Input: part model. Units: mm. Frame: model coordinates. Face numbers are marked on the shaded views. A direction names the side the tool comes from. Round coordinates to 2 decimals unless told otherwise and drop trailing zeros. Order: outer loops, then holes, each group sorted by start corner. A loop starts at its lowest first (then second) coordinate and runs counter-clockwise, first axis right, second up.
Item 1: Cut plane A-A on z = 0. Output: boundary loops of the cut face in (x, y), then the cut area to 3 significant figures.
Item 2: First-contact query: pin 1 (2 mm diameter, centred on x = -1.5, y = 1.5, fed in from +Z). Flat tip, straight axial feed; report the tip coordinate or a pass-through.
Item 3: Cut plane B-B on x = 0. Output: boundary loops of the cut face in (y, z), then the cut area to 3 significant figures.
Item 4: Reachability of the marked faces 1 and 2 from +Z, -Z, +X, -X, +Y, -Y: full face, straight path, thin tool, end or side. Return the list, or none.
Item 5: Cut plane C-C on y = 2. Output: boundary loops of the cut face in (x, z) (1 decimal).
Item 6: Line query: L1, parallel to Y at x = 4.5, z = -5.25; L2, parallel to X at y = 3.25, z = -4.25; L3, parallel to X at y = 2, z = 2.75. Output: solid intervals per line, ascending.
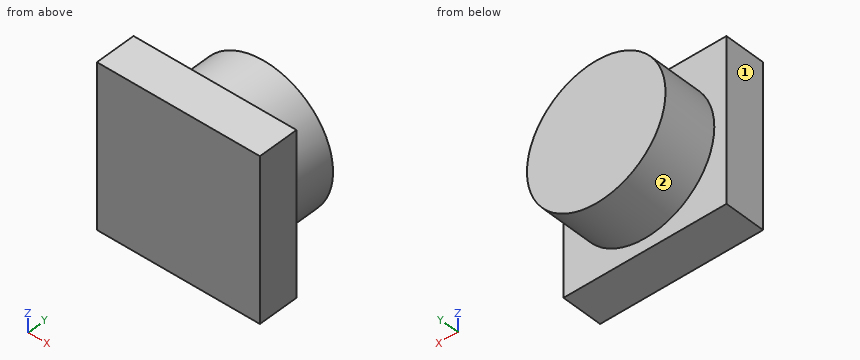
Autodesk Fusion 360 part; units mm, degrees
sketch "Boceto1" plane through (0, 0, 0) normal (0, 1, 0) x (1, 0, 0)
  line L0 (6, 6) -> (-6, 6)
  line L1 (-6, 6) -> (-6, -6)
  line L2 (-6, -6) -> (6, -6)
  line L3 (6, -6) -> (6, 6)
  line L4 (6, 6) -> (-6, -6) construction
  line L5 (-6, 6) -> (6, -6) construction
  circle A0 centre (0, 0) radius 5.1025
  dimension "d2" = 12
  dimension "d3" = 12
extrude "Extruir1" add sketch "Boceto1" along normal blind 4 contours A0
extrude "Extruir2" add sketch "Boceto1" against normal blind 3 contours L0 L1 L2 L3 | A0
From the geometry:
1. outline: (-6, -3) - (6, -3) - (6, 0) - (5.1, 0) - (5.1, 4) - (-5.1, 4) - (-5.1, 0) - (-6, 0) - close
1. area: 76.8 mm2
2. pin 1: stops at z = 5.08
3. outline: (-3, -6) - (0, -6) - (0, -5.1) - (4, -5.1) - (4, 5.1) - (0, 5.1) - (0, 6) - (-3, 6) - close
3. area: 76.8 mm2
4. face 1: +Z, -Z, -X, +Y, -Y
4. face 2: +Y
5. outline: circle Ø10.2 at (0, 0)
6. L1: y = -3 to 0
6. L2: x = -2.82 to 2.82
6. L3: x = -4.3 to 4.3
